Here's how the part is built. I have some questions about the finished solid (model axes, mm). A direction names the side the tool comes from. Give positions to 0.01 mm unless a question says otherwise; leave off trailing zeros. Write each loop counter-clockwise with the first axis right and the second up, starting at its lowest first coordinate (ties: lowest second). Pieces come first, ordered by that corner, then holes. Notation, with made-up numbers: (-1, -29) -> (11, -29) arc R25 ccw to (11, 8) -> close; hole circle Ø5 at (-25.75, 30). An arc over 180 degrees is marked (long way). Answer as CSV lines item,"result". Start each with the question number.
from build123d import *

# Parameters (mm, degrees)
CYLINDER007_R     = 1
CYLINDER007_DEPTH = 20
CYLINDER006_R     = 1
CYLINDER006_DEPTH = 20
CYLINDER008_R     = 1
CYLINDER008_DEPTH = 20
CYLINDER004_R     = 1
CYLINDER004_DEPTH = 20
CYLINDER003_R     = 1
CYLINDER003_DEPTH = 20
CYLINDER005_R     = 1
CYLINDER005_DEPTH = 20
CYLINDER001_R     = 1
CYLINDER001_DEPTH = 20
CYLINDER_R        = 1
CYLINDER_DEPTH    = 20
CYLINDER002_R     = 1
CYLINDER002_DEPTH = 20
BOX001_W          = 12
BOX001_H          = 12
BOX001_DEPTH      = 9
BOX_W             = 13
BOX_H             = 13
BOX_DEPTH         = 10
BOX002_W          = 11
BOX002_H          = 5
BOX002_DEPTH      = 3.5


with BuildPart() as cilindro007:
    # Cylinder007 → Cylinder007 (new body)
    with BuildSketch(Plane(origin=(3.7, 17, 1.2), x_dir=(1, 0, 0), z_dir=(0, -1, 0))):
        Circle(CYLINDER007_R)
    extrude(amount=CYLINDER007_DEPTH)


with BuildPart() as cilindro006:
    # Cylinder006 → Cylinder006 (new body)
    with BuildSketch(Plane(origin=(10.3, 17.7, 1.2), x_dir=(1, 0, 0), z_dir=(0, -1, 0))):
        Circle(CYLINDER006_R)
    extrude(amount=CYLINDER006_DEPTH)


with BuildPart() as cilindro008:
    # Cylinder008 → Cylinder008 (new body)
    with BuildSketch(Plane(origin=(7, 17.7, 1.2), x_dir=(1, 0, 0), z_dir=(0, -1, 0))):
        Circle(CYLINDER008_R)
    extrude(amount=CYLINDER008_DEPTH)


with BuildPart() as cilindro004:
    # Cylinder004 → Cylinder004 (new body)
    with BuildSketch(Plane(origin=(3.7, 1.5, 12), x_dir=(1, 0, 0), z_dir=(0, 0, -1))):
        Circle(CYLINDER004_R)
    extrude(amount=CYLINDER004_DEPTH)


with BuildPart() as cilindro003:
    # Cylinder003 → Cylinder003 (new body)
    with BuildSketch(Plane(origin=(10.3, 1.5, 12), x_dir=(1, 0, 0), z_dir=(0, 0, -1))):
        Circle(CYLINDER003_R)
    extrude(amount=CYLINDER003_DEPTH)


with BuildPart() as cilindro005:
    # Cylinder005 → Cylinder005 (new body)
    with BuildSketch(Plane(origin=(7, 1.5, 12), x_dir=(1, 0, 0), z_dir=(0, 0, -1))):
        Circle(CYLINDER005_R)
    extrude(amount=CYLINDER005_DEPTH)


with BuildPart() as cilindro001:
    # Cylinder001 → Cylinder001 (new body)
    with BuildSketch(Plane(origin=(7, 11.5, 12.2), x_dir=(1, 0, 0), z_dir=(0, 0, -1))):
        Circle(CYLINDER001_R)
    extrude(amount=CYLINDER001_DEPTH)


with BuildPart() as cilindro:
    # Cylinder → Cylinder (new body)
    with BuildSketch(Plane(origin=(3.7, 11.5, 12), x_dir=(1, 0, 0), z_dir=(0, 0, -1))):
        Circle(CYLINDER_R)
    extrude(amount=CYLINDER_DEPTH)


with BuildPart() as cilindro002:
    # Cylinder002 → Cylinder002 (new body)
    with BuildSketch(Plane(origin=(10.3, 11.5, 12), x_dir=(1, 0, 0), z_dir=(0, 0, -1))):
        Circle(CYLINDER002_R)
    extrude(amount=CYLINDER002_DEPTH)


with BuildPart() as cubo001:
    # Box001 → Box001 (new body)
    with BuildSketch(Plane(origin=(0.5, 0.5, 1), x_dir=(1, 0, 0), z_dir=(0, 0, 1))):
        with Locations((6, 6)):
            Rectangle(BOX001_W, BOX001_H)
    extrude(amount=BOX001_DEPTH)


with BuildPart() as cut009:
    # Box → Box (new body)
    with BuildSketch(Plane.XY):
        with Locations((6.5, 6.5)):
            Rectangle(BOX_W, BOX_H)
    extrude(amount=BOX_DEPTH)

    # Cut: cut Cubo001
    add(cubo001.part, mode=Mode.SUBTRACT)

    # Cut001: cut Cilindro002
    add(cilindro002.part, mode=Mode.SUBTRACT)

    # Cut002: cut Cilindro
    add(cilindro.part, mode=Mode.SUBTRACT)

    # Cut003: cut Cilindro001
    add(cilindro001.part, mode=Mode.SUBTRACT)

    # Cut004: cut Cilindro005
    add(cilindro005.part, mode=Mode.SUBTRACT)

    # Cut005: cut Cilindro003
    add(cilindro003.part, mode=Mode.SUBTRACT)

    # Cut006: cut Cilindro004
    add(cilindro004.part, mode=Mode.SUBTRACT)

    # Cut007: cut Cilindro008
    add(cilindro008.part, mode=Mode.SUBTRACT)

    # Cut008: cut Cilindro006
    add(cilindro006.part, mode=Mode.SUBTRACT)

    # Cut009: cut Cilindro007
    add(cilindro007.part, mode=Mode.SUBTRACT)


with BuildPart() as normal:
    # Box002 → Box002 (new body)
    with BuildSketch(Plane(origin=(1, 3.75, -3), x_dir=(1, 0, 0), z_dir=(0, 0, 1))):
        with Locations((5.5, 2.5)):
            Rectangle(BOX002_W, BOX002_H)
    extrude(amount=BOX002_DEPTH)

    # Fusion: union Cut009
    add(cut009.part)


with BuildPart() as normal_1:
    # Fusion placement: moved
    add(normal.part.moved(Location((50, 0, 0))))


solid = normal_1.part
Item 1: We'd pull the mould along Z, two halves only. Please class faces 6 (the face through (60.76, 12.65, 0.31)), 7 (the face through (61.231, 6.567, 0.836)), 8 (the face through (60.76, 0.37, 0.31)), 9 (the face through (50.5, 6, 5)): released by +Z, released by -Z, zero draft, split by the parting line, or undercut.
Item 2: If we section it at B-B (z = 2.75): Please give me the cut outline in (x, y).
Item 3: If we section it at A-A (x = 53.7): Please give me the cut outline in (y, z).
Item 4: If I drill on line 1 (X direction, y = 1.5, z = 0.7); line 2 (Y direction, x = 53.5, z = 6.5); line 3 (X direction, y = 9, z = 7.75), over which ranges is the centre line in solid material (lowest first)? Write a range as [from, to].
Item 5: If we section it at D-D (z = 1.2): State how many separate pieces and enclosed holes the cut face has, and give its area (3 significant figures).
Item 6: For faces 1 (the face through (62.5, 6, 5)), 2 (the face through (62, 6, -2)), 3 (the face through (57.46, 0.37, 0.31)), 4 (the face through (56, 3.75, -2)), 5 (the face through (54, 6, 0.5)), which set-ups out of +Z, -Z, +X, -X, +Y, -Y let a thin tool reach every point of the face, with its end or its side?
Item 7: If we section it at C-C (y = 1.5): Please give me the cut outline in (x, z).
Item 8: I'm going to push flat-ended pins straight in: pin 1 (2.5 mm diameter, centred on x = 60.3, y = 1.5, fed in from +Z); pin 2 (1.6 mm diameter, centred on x = 60.3, z = 1.2, fed in from -Y); pin 3 (5 mm diameter, centred on x = 57.5, y = 5, fed in from +Z); pin 4 (1.2 mm diameter, centred on x = 57, y = 1.5, fed in from +Z). Where does each tip first touch, or does it pass through?
Final values:
1,face 6,"undercut"
1,face 7,"released by +Z"
1,face 8,"undercut"
1,face 9,"zero draft"
2,outline,"(50, 0) -> (63, 0) -> (63, 13) -> (50, 13) -> close; hole (50.5, 0.5) -> (62.5, 0.5) -> (62.5, 12.5) -> (50.5, 12.5) -> close"
3,outline,"(0, 0) -> (0.5, 0) -> (0.5, 0.2) -> (0, 0.2) -> close; (0, 2.2) -> (0.5, 2.2) -> (0.5, 10) -> (0, 10) -> close; (2.5, 0) -> (3.75, 0) -> (3.75, -3) -> (8.75, -3) -> (8.75, 0) -> (10.5, 0) -> (10.5, 0.2) -> (8.75, 0.2) -> (8.75, 0.5) -> (3.75, 0.5) -> (3.75, 0.2) -> (2.5, 0.2) -> close; (12.5, 0) -> (13, 0) -> (13, 0.2) -> (12.5, 0.2) -> close; (12.5, 2.2) -> (13, 2.2) -> (13, 10) -> (12.5, 10) -> close"
4,line 1,"[50, 52.7], [54.7, 56], [58, 59.3], [61.3, 63]"
4,line 2,"[0, 0.5], [12.5, 13]"
4,line 3,"[50, 50.5], [62.5, 63]"
5,separate pieces,"6"
5,enclosed holes,"0"
5,area,"19.0 mm2"
6,face 1,"+Z"
6,face 2,"-Z, +X, +Y, -Y"
6,face 3,"-Y"
6,face 4,"-Z, +X, -X, -Y"
6,face 5,"+Z, +Y, -Y"
7,outline,"(50, 0) -> (52.7, 0) -> (52.7, 1) -> (50.5, 1) -> (50.5, 10) -> (50, 10) -> close; (54.7, 0) -> (56, 0) -> (56, 1) -> (54.7, 1) -> close; (58, 0) -> (59.3, 0) -> (59.3, 1) -> (58, 1) -> close; (61.3, 0) -> (63, 0) -> (63, 10) -> (62.5, 10) -> (62.5, 1) -> (61.3, 1) -> close"
8,pin 1,"z = 10"
8,pin 2,"y = 3.75"
8,pin 3,"z = 1"
8,pin 4,"through"
